```python
from build123d import *

# Parameters (mm, degrees)
F0_W     = 44
F0_H     = 99
F1_DEPTH = 20
F2_R     = 10
F4_DEPTH = 3
F5_SIZE2 = 1.5
F5_SIZE  = 6
F6_R     = 10
F7_DEPTH = 1
F8_R     = 4.5
F9_DEPTH = 1


with BuildPart() as f1:
    # F0 (on Top) → F1 (new body)
    with BuildSketch(Plane.XY):
        Rectangle(F0_W, F0_H)
    extrude(amount=F1_DEPTH)

    # F2
    f2_edges = [f1.edges().sort_by_distance(p)[0] for p in [
        (22, 49.5, 10),
        (-22, -49.5, 10),
    ]]
    fillet(f2_edges, radius=F2_R)

    # F3 (on face) → F4 (join)
    with BuildSketch(Plane.XY.offset(20)):
        with BuildLine():
            ThreePointArc((24, 39.5), (20.4852813742, 47.9852813742), (12, 51.5))
            Line((12, 51.5), (-24, 51.5))
            Line((-24, 51.5), (-24, -39.5))
            ThreePointArc((-24, -39.5), (-20.4852813742, -47.9852813742), (-12, -51.5))
            Line((-12, -51.5), (24, -51.5))
            Line((24, -51.5), (24, 39.5))
        make_face()
    extrude(amount=-F4_DEPTH)

    # F5
    f5_edges = [f1.edges().sort_by_distance(p)[0] for p in [
        (20.485281, 47.985281, 20),
        (-6, 51.5, 20),
        (-24, 6, 20),
        (-20.485281, -47.985281, 20),
        (6, -51.5, 20),
        (24, -6, 20),
    ]]
    f5_side = f1.faces().sort_by_distance((0, 0, 20))[0]
    chamfer(f5_edges, length=F5_SIZE, length2=F5_SIZE2, reference=f5_side)

    # F6 (on face) → F7 (cut)
    with BuildSketch(Plane.XY.offset(20)):
        with Locations((0, 26.5)):
            Circle(F6_R)
    extrude(amount=-F7_DEPTH, mode=Mode.SUBTRACT)

    # F8 (on face) → F9 (cut)
    with BuildSketch(Plane(origin=(0, 0, 0), x_dir=(1, 0, 0), z_dir=(0, 0, -1))):
        Circle(F8_R)
        with BuildLine():
            Line((-2, -32), (-2, -37))
            ThreePointArc((-2, -37), (0, -39), (2, -37))
            Line((2, -37), (2, -32))
            ThreePointArc((2, -32), (0, -30), (-2, -32))
        make_face()
        with BuildLine():
            Line((2.5, 36.5), (-2.5, 36.5))
            ThreePointArc((-2.5, 36.5), (-4.5, 34.5), (-2.5, 32.5))
            Line((-2.5, 32.5), (2.5, 32.5))
            ThreePointArc((2.5, 32.5), (4.5, 34.5), (2.5, 36.5))
        make_face()
    extrude(amount=-F9_DEPTH, mode=Mode.SUBTRACT)


solid = f1.part
```
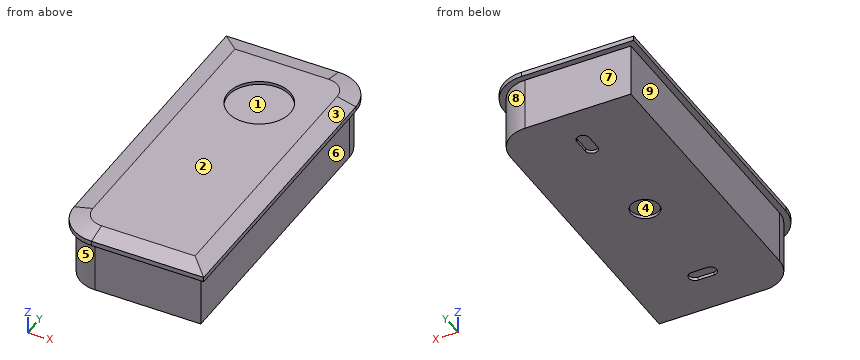
Geometry check sheet. Reference: the model listing, model coordinates, mm. Face numbers are marked on the shaded views. A direction names the side the tool comes from. Give positions to 0.01 mm unless a question says otherwise; leave off trailing zeros. Loops run counter-clockwise (first coordinate to the right, second up) from the corner with the lowest first, then second, coordinate; pieces in that order, holes last. Notation, with made-up numbers: M -2.5,-3.5 L 50.5,-3.5 A20 cw 50.5,21.5 Z; hole C -21,-1.75 d8. An arc over 180 degrees is marked long. Write item = value, one per line. Start each with the question number.
1. Thickness scan on probe 1 along Y at (x, z) = (0, 0.3); probe 2 along X at (y, z) = (0, 0.7); probe 3 along Z at (x, y) = (-6, 24). Record the ranges inside material, lowest first.
2. Section check D-D, the plane y = 0. Enter the section's corners in (x, z), plus the area to 3 significant figures.
3. Tool access check on the marked faces 5, 6, 7, 8 and 9. Record the directions out of +Z, -Z, +X, -X, +Y, -Y that give a thin tool (end or side, any length) a straight path to the whole face; none if there is none.
4. Section check C-C, the plane z = 14.25. Enter the section's corners in (x, y), plus the area to 3 significant figures.
5. Section check A-A, the plane y = 26.5. Enter the section's corners in (x, z), plus the area to 3 significant figures.
6. Go/stop test with flat-tipped pins: P1, Ø1.1, axis at x = -1, z = 0.5, coming from the +Y side; P2, Ø4, axis at y = -0.5, z = 7, coming from the -X side; P3, Ø12, axis at x = 0, y = 26.5, coming from the +Z side. Record where each tip stops, or that it passes through.
7. Draft check along X on the marked faces 1, 2, 3 and 4. Enter one of: +X half, -X half, draft (parallel to the pull), parting line (faces both ways), or undercut.
8. Section check B-B, the plane x = 0. Enter the section's corners in (y, z).
Values follow:
q1.probe_1 = -49.5 to -36.5, -32.5 to -4.5, 4.5 to 30, 39 to 49.5
q1.probe_2 = -22 to -4.5, 4.5 to 22
q1.probe_3 = 0 to 19
q2.outline = M -24,17 L -22,17 L -22,0 L -4.5,0 L -4.5,1 L 4.5,1 L 4.5,0 L 22,0 L 22,17 L 24,17 L 24,18.5 L 18,20 L -18,20 L -24,18.5 Z
q2.area = 874 mm^2
q3.face_5 = -Z, -X, -Y
q3.face_6 = -Z, +X, +Y, -Y
q3.face_7 = -Z, +X, -X, +Y
q3.face_8 = -Z, +X, +Y
q3.face_9 = -Z, -X, +Y, -Y
q4.outline = M -22,-39.5 A10 ccw -12,-49.5 L 22,-49.5 L 22,39.5 A10 ccw 12,49.5 L -22,49.5 Z
q4.area = 4,310 mm^2
q5.outline = M -24,17 L -22,17 L -22,0 L 22,0 L 22,17 L 24,17 L 24,18.5 L 18,20 L 10,20 L 10,19 L -10,19 L -10,20 L -18,20 L -24,18.5 Z
q5.area = 863 mm^2
q6.P1 = 49.5
q6.P2 = -22
q6.P3 = 19
q7.face_1 = undercut
q7.face_2 = draft
q7.face_3 = +X half
q7.face_4 = undercut
q8.outline = M -51.5,17 L -49.5,17 L -49.5,0 L -36.5,0 L -36.5,1 L -32.5,1 L -32.5,0 L -4.5,0 L -4.5,1 L 4.5,1 L 4.5,0 L 30,0 L 30,1 L 39,1 L 39,0 L 49.5,0 L 49.5,17 L 51.5,17 L 51.5,18.5 L 45.5,20 L 36.5,20 L 36.5,19 L 16.5,19 L 16.5,20 L -45.5,20 L -51.5,18.5 Z
